Design review of the part shown in the three views and the two pictorial views. Dimensions are in mm from the part's minimum x, y and z. Coordinates: 2 decimals unless noted, no trailing zeros. Order: outer loops, then holes, each group sorted by start corner. A loop starts at its lowest first (then second) coordinate and runs counter-clockwise, first axis right, second up. Notation, with made-up numbers: (40, -23) -> (50, -23) arc R24 cw to (50, 4) -> close; hole circle Ø6 at (13, 31.25). An arc over 180 degrees is marked (long way). Answer as a JSON object with one key per item and string values. Group by question number.
1) Draft analysis for pull direction Z (two halves, no side actions). For the marked faces 1, 2 and 3, state which applies: +Z half, -Z half, draft (parallel to the pull), parting line (faces both ways), or undercut.
2) Add section C-C, the plane y = 1.05. Write out the cut boundary in (x, z).
3) Add section A-A, the plane x = 2. Write out the cut boundary in (y, z), then the cut area to 3 significant figures.
4) Add section B-B, the plane z = 2.9. Write out the cut boundary in (x, y).
5) For pin 1 (0.7 mm diameter, centred on x = 2, z = 2.9, fed in from -Y), flat-tipped, find the tip position at first contact; note if it passes through.
6) Wall thickness on L1, parallel to Z at x = 13, y = 0.85; L2, parallel to X at y = 0.7, z = 2.5; L3, parallel to X at y = 0.25, z = 3: over which ranges is each line inside the solid? List them lowest first.
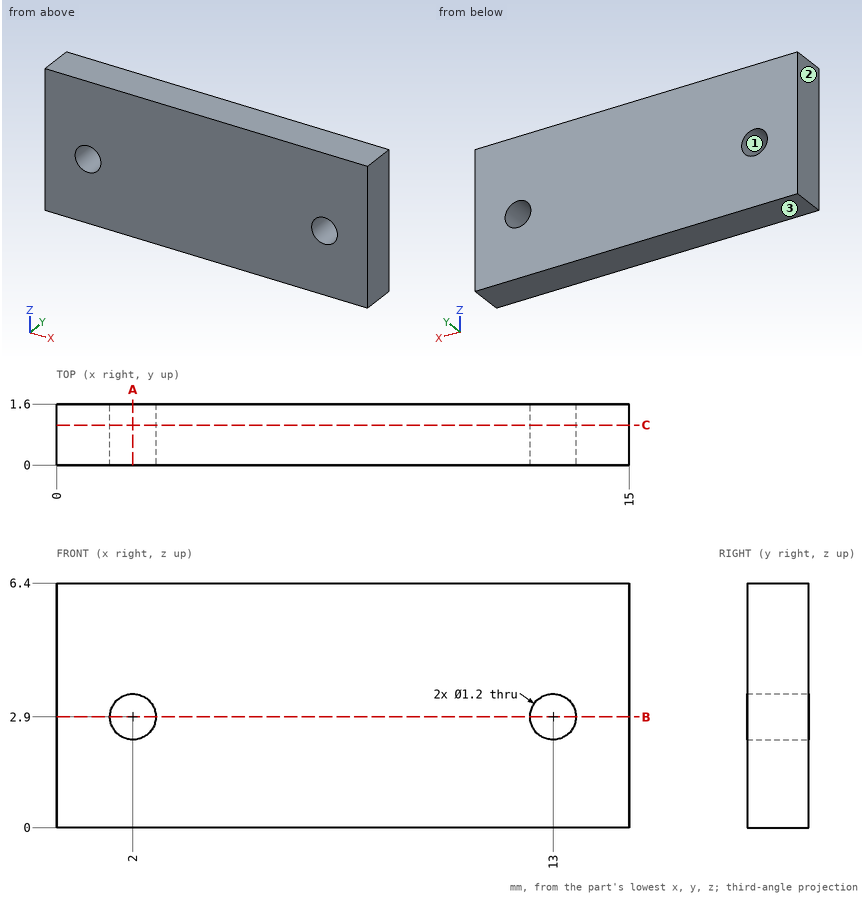
Output values:
{
 "1": {"face 1": "undercut", "face 2": "draft", "face 3": "-Z half"},
 "2": {"outline": "(0, 0) -> (15, 0) -> (15, 6.4) -> (0, 6.4) -> close; hole circle Ø1.2 at (2, 2.9); hole circle Ø1.2 at (13, 2.9)"},
 "3": {"outline": "(0, 0) -> (1.6, 0) -> (1.6, 2.3) -> (0, 2.3) -> close; (0, 3.5) -> (1.6, 3.5) -> (1.6, 6.4) -> (0, 6.4) -> close", "area": "8.32 mm²"},
 "4": {"outline": "(0, 0) -> (1.4, 0) -> (1.4, 1.6) -> (0, 1.6) -> close; (2.6, 0) -> (12.4, 0) -> (12.4, 1.6) -> (2.6, 1.6) -> close; (13.6, 0) -> (15, 0) -> (15, 1.6) -> (13.6, 1.6) -> close"},
 "5": {"pin 1": "passes through"},
 "6": {"L1": "z = 0 to 2.3, 3.5 to 6.4", "L2": "x = 0 to 1.55, 2.45 to 12.55, 13.45 to 15", "L3": "x = 0 to 1.41, 2.59 to 12.41, 13.59 to 15"}
}
